Autodesk Inventor part; units mm, degrees
ref_plane "YZ Plane" through (0, 0, 0) normal (1, 0, 0) x (0, 1, 0)
ref_plane "XZ Plane" through (0, 0, 0) normal (0, 1, 0) x (-1, 0, 0)
ref_plane "XY Plane" through (0, 0, 0) normal (0, 0, 1) x (1, 0, 0)
sketch "Sketch1" plane through (0, 0, 0) normal (0, 0, 1) x (1, 0, 0)
  circle A0 centre (0, 0) radius 195 construction
  line L0 (0, 195) -> (0, 225) construction
  line L1 (0, 195) -> (0, 165) construction
  circle A1 centre (0, 0) radius 165
  circle A2 centre (0, 0) radius 225
  line L2 (-165, 0) -> (-165, 80)
  line L3 (-165, 80) -> (-225, 80)
  line L4 (-225, 80) -> (-225, 0)
  line L5 (165, 0) -> (165, 80)
  line L6 (165, 80) -> (225, 80)
  line L7 (225, 80) -> (225, 0)
  line L8 (-225, 0) -> (-165, 0)
  line L9 (165, 0) -> (225, 0)
  line L10 (-225, 0) -> (-285, 0)
  line L11 (-285, 0) -> (-285, -50)
  line L12 (-285, -50) -> (-219.3741, -50)
  line L13 (225, 0) -> (285, 0)
  line L14 (285, 0) -> (285, -50)
  line L15 (285, -50) -> (219.3741, -50)
  dimension "d13" = 390
  dimension "d26" = 80
  dimension "d36" = 60
  dimension "d40" = 60
  dimension "d41" = 50
extrude "Extrusion1" add sketch "Sketch1" against normal blind 30 contours L9 A2 L8 A1 | L13 L14 L15 A2 | A2 L12 L11 L10
sketch "Sketch7" plane through (-285, 0, 0) normal (0, 1, 0) x (1, 0, 0)
  circle A0 centre (25, 15) radius 7
  line L0 (0, 0) -> (0, 30)
  point P0 (285, 0)
  point P1 (0, 15)
  dimension "d42" = 14
  dimension "d43" = 25
extrude "Extrusion7" cut sketch "Sketch7" against normal through all
mirror "Mirror1" about plane through (0, 0, 0) normal (1, 0, 0) of "Extrusion7"
equation "\"d13\" = Шпил_пласт_НОС_диам_центров"
equation "\"d40\" = d36"
equation "\"BendReliefDepth\" = 0.5 * Thickness"
properties part number "ДМФ 092 Коромысло НОС"
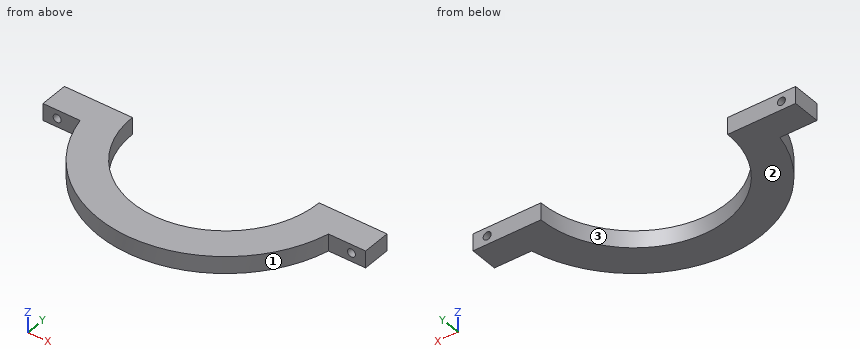
The model under review builds one solid part; all positions refer to its coordinate system, in mm. Face numbers are marked on the shaded views. Coordinates: 2 decimals unless noted, no trailing zeros. Loops run counter-clockwise (first coordinate to the right, second up) from the corner with the lowest first, then second, coordinate; pieces in that order, holes last. Notation, with made-up numbers: (-31, 77) -> (-18, 77) arc R7 ccw to (-18, 82) -> close; hole circle Ø2 at (63, -5). An arc over 180 degrees is marked (long way). Use a Markdown table: item, result. Add a question column.
1. Add section C-C on z = -15. Write out the cut boundary in (x, y), plus the area to 3 significant figures.
2. Add section B-B on x = -260. Write out the cut boundary in (y, z).
3. Draft analysis for pull direction X (two halves, no side actions). For the marked faces 1, 2 and 3, state which applies: pulls with the +X half, pulls with the -X half, needs draft (parallel to the pull), parting line crosses it, or undercut.
4. To check wall thickness, follow line 1 (Z direction, x = 260, y = -23); line 2 (X direction, y = -19.5, z = -15); line 3 (X direction, y = -13, z = -16.25). State the ranges of each line that lie inside material, in increasing order.
5. Add section A-A on y = -28.5. Write out the cut boundary in (x, z).
6. Clearance check with flat-ended pins moving along their axes: pin 1 Ø6 at (y, z) = (-197.5, -9) entering from +X; pin 2 Ø8 at (y, z) = (-133.5, -12.5) entering from +X; pin 3 Ø5 at (y, z) = (-115, -9.5) entering from +X; pin 4 Ø12 at (x, y) = (43.5, -161) entering from +Z. State where each tip first meets the part, or that it passes through.
7. Add section D-D on y = -85.5. Write out the cut boundary in (x, z), plus the area to 3 significant figures.
Returned:
| question | item | result |
|---|---|---|
| 1 | outline | (-285, -50) -> (-267, -50) -> (-267, 0) -> (-285, 0) -> close; (-253, -50) -> (-219.37, -50) arc R225 ccw to (219.37, -50) -> (253, -50) -> (253, 0) -> (165, 0) arc R165 cw to (-165, 0) -> (-253, 0) -> close; (267, -50) -> (285, -50) -> (285, 0) -> (267, 0) -> close |
| 1 | area | 41,500 mm² |
| 2 | outline | (-50, -30) -> (0, -30) -> (0, -22) -> (-50, -22) -> close; (-50, -8) -> (0, -8) -> (0, 0) -> (-50, 0) -> close |
| 3 | face 1 | parting line crosses it |
| 3 | face 2 | needs draft |
| 3 | face 3 | undercut |
| 4 | line 1 | z = -30 to -22, -8 to 0 |
| 4 | line 2 | x = -285 to -267, -253 to -163.84, 163.84 to 253, 267 to 285 |
| 4 | line 3 | x = -285 to -266.89, -253.11 to -164.49, 164.49 to 253.11, 266.89 to 285 |
| 5 | outline | (-285, -30) -> (-162.52, -30) -> (-162.52, 0) -> (-285, 0) -> close; (162.52, -30) -> (285, -30) -> (285, 0) -> (162.52, 0) -> close; hole circle Ø14 at (-260, -15); hole circle Ø14 at (260, -15) |
| 6 | pin 1 | stops at x = 113.11 |
| 6 | pin 2 | stops at x = 184 |
| 6 | pin 3 | stops at x = 194.86 |
| 6 | pin 4 | stops at z = 0 |
| 7 | outline | (-208.12, -30) -> (-141.12, -30) -> (-141.12, 0) -> (-208.12, 0) -> close; (141.12, -30) -> (208.12, -30) -> (208.12, 0) -> (141.12, 0) -> close |
| 7 | area | 4,020 mm² |
